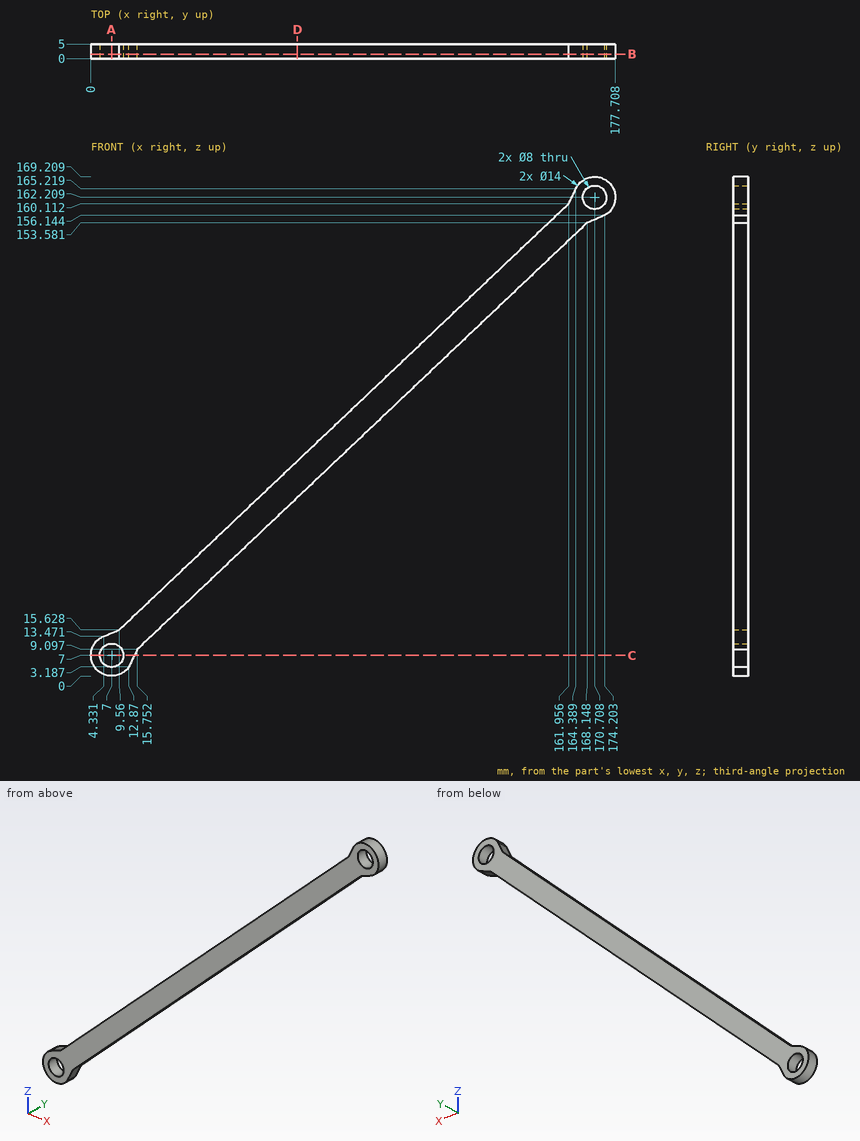
Geometry: see drawing. Coordinates: mm, zero at the bounding-box minimum. Give positions to 0.01 mm unless a question says otherwise; leave off trailing zeros. Order: outer loops, then holes, each group sorted by start corner. A loop starts at its lowest first (then second) coordinate and runs counter-clockwise, first axis right, second up. Notation, with made-up numbers: (74.5, -22) - (132.5, -22) arc R20 ccw to (132.5, -10) - close; hole circle Ø9 at (-12.5, 14.5). An arc over 180 degrees is marked (long way). Write each question's results on one line, items separated by ' | '.
Item 1: Section D-D (x = 70). Return loops of the section in (y, z), and give its area (3 significant figures).
A:
outline: (0, 60.53) - (5, 60.53) - (5, 72.93) - (0, 72.93) - close | area: 62.0 mm^2
Item 2: Section C-C (z = 7). Return loops of the section in (x, y).
A:
outline: (0, 0) - (3, 0) - (3, 5) - (0, 5) - close; (11, 0) - (14.73, 0) - (14.73, 5) - (11, 5) - close
Item 3: Material intervals for line 1 along Z through (x, y) = (7, 1.55); line 2 along X through (y, z) = (3.2, 7); line 3 along Z through (x, y) = (24, 0.35) (1 decimal), sorted ascending.
A:
line 1: z = 0 to 3, 11 to 14.57 | line 2: x = 0 to 3, 11 to 14.73 | line 3: z = 16.9 to 29.3
Item 4: Section B-B (y = 1.6). Return loops of the section in (x, z).
A:
outline: (4.33, 13.47) arc R7 ccw (long way) to (12.87, 3.19) - (15.75, 9.1) - (168.15, 153.58) - (174.2, 156.14) arc R7 ccw (long way) to (164.39, 165.22) - (161.96, 160.11) - (9.56, 15.63) - close; hole circle Ø8 at (7, 7); hole circle Ø8 at (170.71, 162.21)
Item 5: Section A-A (x = 7). Return loops of the section in (y, z).
A:
outline: (0, 0) - (5, 0) - (5, 3) - (0, 3) - close; (0, 11) - (5, 11) - (5, 14.57) - (0, 14.57) - close
Item 6: Contact query for flat-ended pins moving along their axis: pin 1 Ø2 at (y, z) = (4, 29.5) entering from -X (1 decimal); pin 2 Ø2 at (y, z) = (3.5, 109) entering from +X; pin 3 Ø1.5 at (y, z) = (1.5, 76) entering from -X (1 decimal). Output: stop coordinate, or through.
A:
pin 1: stops at x = 23.1 | pin 2: stops at x = 122.18 | pin 3: stops at x = 72.4
